Input: part model. Units: mm. Frame: model coordinates. A direction names the side the tool comes from. Round coordinates to 2 decimals unless told otherwise and drop trailing zeros. Loops run counter-clockwise (first coordinate to the right, second up) from the corner with the lowest first, then second, coordinate; pieces in that order, holes last. Notation, with made-up numbers: (34, 8.25) -> (46, 8.25) arc R16 ccw to (46, 39.25) -> close; hole circle Ø7 at (-29, 10). An arc over 180 degrees is marked (long way). Answer as a JSON object with one key per item and string values. Group by question number.
Item 1: Set-up query: faces 1 (the flat face through (0, 21.2, 0)), 2 (the cylindrical face through (0.29, 9.85, -2.23)). Return all of +Z, -Z, +X, -X, +Y, -Y with unobstructed straight access to the full face (end or side cutting, diameter ignored); none if empty.
Item 2: Section query D-D on x = 11.75. Return loops of the section in (y, z).
Item 3: Pin query (flat end, axial travel): pin 1 (12 mm diameter, centred on x = -1.5, y = 12.5, fed in from -Z) (3 decimals); pin 2 (2 mm diameter, centred on x = -1, z = 0, fed in from -Y); pin 3 (12 mm diameter, centred on y = 19, z = 3.5, fed in from -X); pin 4 (3 mm diameter, centred on x = -9.5, y = 17.5, fed in from -Z). Return the tip coordinate at first contact, or that it passes through.
Item 4: Draft query along Z for faces 3 (the flat face through (4, 22, 6)), 4 (the flat face through (2.812, 11.644, -4.136)). Return one class per face: released by +Z, released by -Z, zero draft, split by the parting line, or undercut.
Item 5: Material intervals for line 1 (Z direction, x = 4, y = 10.5); line 2 (Z direction, x = -8, y = 10.5); line 3 (X direction, y = 12, z = 5), sorted ascending. Write a range as [from, to].
Item 6: Section query B-B on y = 4.5. Return loops of the section in (x, z), and give its area (3 significant figures).
Item 7: Section query A-A on x = 0. Return loops of the section in (y, z), and give its area (3 significant figures).
Item 8: Section query C-C on y = 20.5. Return loops of the section in (x, z), and give its area (3 significant figures).
from build123d import *

# Parameters (mm, degrees)
REVOLVE2_ANGLE                       = 180
BOSS_EXTRUDE4_REACH                  = 31.155
BOSS_EXTRUDE4_END_RADIUS             = 15
SKETCH6_R                            = 2.25
SKETCH7_R                            = 10
BOSS_EXTRUDE6_DEPTH                  = 2
BOSS_EXTRUDE6_TAPER                  = 45
SKETCH8_R                            = 7
CUT_EXTRUDE1_DEPTH                   = 0.8
CUT_EXTRUDE1_DRAFT                   = -60
SKETCH3_W                            = 2.2
SKETCH3_H                            = 1.5
CUT_EXTRUDE4_DEPTH                   = 8
BOSS_EXTRUDE7_REACH                  = 28.571
BOSS_EXTRUDE7_END_RADIUS             = 14
SKETCH10_R                           = 2.25
SKETCH10_W                           = 2.2
SKETCH10_H                           = 1.5
BOSS_EXTRUDE9_REACH                  = 33.726
BOSS_EXTRUDE9_END_RADIUS             = 14
SKETCH12_W                           = 0.734734754
SKETCH12_H                           = 3.5
BOSS_EXTRUDE9_DIRECTION_2_REACH      = 33.726
BOSS_EXTRUDE9_DIRECTION_2_END_RADIUS = 2.25
CIRPATTERN1_COUNT                    = 6


with BuildPart() as part:
    # Sketch1 → Revolve2 (revolve)
    with BuildSketch(Plane(origin=(0, 0, 0), x_dir=(1, 0, 0), z_dir=(0, 1, 0))):
        with BuildLine():
            Line((0, -14), (0, -15))
            ThreePointArc((0, -15), (-15, 0), (0, 15))
            Line((0, 15), (0, 14))
            ThreePointArc((0, 14), (-14, 0), (0, -14))
        make_face()
    revolve(axis=Axis((0, 0, -14), (0, 0, -1)), revolution_arc=REVOLVE2_ANGLE)

    # Boss-Extrude4: up to this sphere (the profile starts outside it)
    boss_extrude4_end = Location((0, 0, 0)) * Sphere(BOSS_EXTRUDE4_END_RADIUS, mode=Mode.PRIVATE)
    # Sketch6 → Boss-Extrude4 (add, up to the surface)
    with BuildSketch(Plane(origin=(0, 20, 0), x_dir=(1, 0, 0), z_dir=(0, 1, 0)), mode=Mode.PRIVATE) as boss_extrude4_sk1:
        with Locations(Location((0, 0, 0), (0, 0, 180))):
            Circle(SKETCH6_R)
    boss_extrude4_tool1 = extrude(boss_extrude4_sk1.sketch, amount=-BOSS_EXTRUDE4_REACH, mode=Mode.PRIVATE) - boss_extrude4_end
    add(boss_extrude4_tool1.solids().sort_by_distance((0, 20, 0))[0])

    # Sketch7 → Boss-Extrude6 (add)
    with BuildSketch(Plane(origin=(0, 20, 0), x_dir=(1, 0, 0), z_dir=(0, 1, 0))):
        Circle(SKETCH7_R)
    extrude(amount=BOSS_EXTRUDE6_DEPTH, taper=BOSS_EXTRUDE6_TAPER)


with BuildPart() as cut_extrude1_tool:
    # Sketch8 → Cut-Extrude1 (with draft: the straight prism first)
    with BuildSketch(Plane(origin=(0, 22, 0), x_dir=(1, 0, 0), z_dir=(0, 1, 0))):
        Circle(SKETCH8_R)
    extrude(amount=-CUT_EXTRUDE1_DEPTH)
    # Cut-Extrude1: the draft: its side faces are tilted about the plane it starts from
    cut_extrude1_sides = [cut_extrude1_tool.faces().sort_by_distance(p)[0] for p in [
        (-7, 21.6, 0),
    ]]
    draft(cut_extrude1_sides, Plane(origin=(0, 22, 0), x_dir=(1, 0, 0), z_dir=(0, 1, 0)), CUT_EXTRUDE1_DRAFT)


with BuildPart() as part_1:
    add(part.part)

    # Cut-Extrude1: cut by cut_extrude1_tool
    add(cut_extrude1_tool.part, mode=Mode.SUBTRACT)

    # Sketch3 → Cut-Extrude4 (cut)
    with BuildSketch(Plane(origin=(0, 6, 0), x_dir=(-1, 0, 0), z_dir=(0, -1, 0))):
        Rectangle(SKETCH3_W, SKETCH3_H)
    extrude(amount=-CUT_EXTRUDE4_DEPTH, mode=Mode.SUBTRACT)

    # Boss-Extrude7: up to this sphere (the profile starts inside it)
    boss_extrude7_end = Location((0, 0, 0)) * Sphere(BOSS_EXTRUDE7_END_RADIUS, mode=Mode.PRIVATE)
    # Sketch10 → Boss-Extrude7 (add, up to the surface)
    with BuildSketch(Plane(origin=(0, 6, 0), x_dir=(-1, 0, 0), z_dir=(0, -1, 0)), mode=Mode.PRIVATE) as boss_extrude7_sk1:
        Circle(SKETCH10_R)
        Rectangle(SKETCH10_W, SKETCH10_H, mode=Mode.SUBTRACT)
    boss_extrude7_tool1 = extrude(boss_extrude7_sk1.sketch, amount=-BOSS_EXTRUDE7_REACH, mode=Mode.PRIVATE) & boss_extrude7_end
    add(boss_extrude7_tool1.solids().sort_by_distance((2.18636, 6, 0))[0])

    # Boss-Extrude9: up to this sphere (the profile starts inside it)
    boss_extrude9_end = Location((0, 0, 0)) * Sphere(BOSS_EXTRUDE9_END_RADIUS, mode=Mode.PRIVATE)
    # Sketch12 → Boss-Extrude9 (add, up to the surface)
    with BuildSketch(Plane.ZY.offset(2.25), mode=Mode.PRIVATE) as boss_extrude9_sk1:
        with Locations((0, 12.057093613)):
            Rectangle(SKETCH12_W, SKETCH12_H)
    boss_extrude9_tool1 = extrude(boss_extrude9_sk1.sketch, amount=BOSS_EXTRUDE9_REACH, mode=Mode.PRIVATE) & boss_extrude9_end
    boss_extrude9 = boss_extrude9_tool1.solids().sort_by_distance((-2.25, 12.057094, 0))[0]
    add(boss_extrude9)

    # Boss-Extrude9 direction 2: up to this cylinder (the profile starts outside it)
    boss_extrude9_direction_2_end = Plane(origin=(0, 12.057094, 0), z_dir=(0, -1, 0)) * Cylinder(BOSS_EXTRUDE9_DIRECTION_2_END_RADIUS, 72.952, mode=Mode.PRIVATE)
    # Sketch12 → Boss-Extrude9 direction 2 (add, up to the surface)
    with BuildSketch(Plane.ZY.offset(2.25), mode=Mode.PRIVATE) as boss_extrude9_direction_2_sk1:
        with Locations((0, 12.057093613)):
            Rectangle(SKETCH12_W, SKETCH12_H)
    boss_extrude9_direction_2_tool1 = extrude(boss_extrude9_direction_2_sk1.sketch, amount=-BOSS_EXTRUDE9_DIRECTION_2_REACH, mode=Mode.PRIVATE) - boss_extrude9_direction_2_end
    boss_extrude9_direction_2 = boss_extrude9_direction_2_tool1.solids().sort_by_distance((-2.25, 12.057094, 0))[0] + boss_extrude9_direction_2_tool1.solids().sort_by_distance((-2.25, 12.057094, 0))[1]
    add(boss_extrude9_direction_2)
    boss_extrude9 = boss_extrude9 + boss_extrude9_direction_2  # both directions under the feature's name, for the pattern or mirror that repeats it

    # CirPattern1: Boss-Extrude9 ×6 about axis
    cirpattern1_axis = Axis((0, 0, 0), (0, 1, 0))
    for i in range(1, CIRPATTERN1_COUNT):
        add(boss_extrude9.rotate(cirpattern1_axis, i * 360 / CIRPATTERN1_COUNT))


solid = part_1.part
Solved:
{
 "1": {"face 1": "+Y", "face 2": "-Y"},
 "2": {"outline": "(0, -9.32) arc R9.32 ccw to (0, 9.32) -> (0, 7.61) arc R7.61 cw to (0, -7.61) -> close"},
 "3": {"pin 1": "z = -13.475", "pin 2": "y = 6", "pin 3": "x = -10", "pin 4": "through"},
 "4": {"face 3": "zero draft", "face 4": "undercut"},
 "5": {"line 1": "[-9.94, -8.35], [-7.66, -6.19], [-0.37, 0.37], [6.19, 7.66], [8.35, 9.94]", "line 2": "[-7.12, -4.66], [-0.37, 0.37], [4.66, 7.12]", "line 3": "[-7.48, -5.2], [-3.31, -2.46], [2.46, 3.31], [5.2, 7.48]"},
 "6": {"outline": "circle Ø28.62 at (0, 0); hole circle Ø26.51 at (0, 0)", "area": "91.1 mm²"},
 "7": {"outline": "(0, -15) arc R15 ccw to (14.83, -2.25) -> (20, -2.25) -> (20, -10) -> (22, -8) -> (22, -7) -> (21.2, -5.61) -> (21.2, 5.61) -> (22, 7) -> (22, 8) -> (20, 10) -> (20, 2.25) -> (14.83, 2.25) arc R15 ccw to (0, 15) -> (0, 14) arc R14 cw to (13.82, 2.25) -> (6, 2.25) -> (6, 0.75) -> (14, 0.75) -> (14, -0.75) -> (6, -0.75) -> (6, -2.25) -> (13.82, -2.25) arc R14 cw to (0, -14) -> close", "area": "118 mm²"},
 "8": {"outline": "circle Ø19 at (0, 0)", "area": "284 mm²"}
}
